```python
from build123d import *

# Parameters (mm, degrees)
ESTRUSIONE_ESTRUSIONE1_DEPTH      = 6
SCHIZZO2_R                        = 2.5
TAGLIO_ESTRUSIONE1_DEPTH          = 3
SCHIZZO3_R                        = 1.75
TAGLIO_ESTRUSIONE2_DEPTH          = 12.513144662
TAGLIO_ESTRUSIONE3_START          = -2
SCHIZZO4_R                        = 2.5
SCHIZZO4_R_2                      = 1.75
TAGLIO_ESTRUSIONE3_DEPTH          = 2
TAGLIO_ESTRUSIONE4_DEPTH          = 5
ESTRUSIONE_ESTRUSIONE2_DEPTH      = 0.2
ESTRUSIONE_ESTRUSIONE2_DEPTH_BACK = 1.2
SCHIZZO5_R                        = 2.25


with BuildPart() as part:
    # Schizzo1 → Estrusione-Estrusione1 (new body)
    with BuildSketch(Plane.XY):
        with BuildLine():
            Line((7.05, -3.5), (-7.05, -3.5))
            ThreePointArc((-7.05, -3.5), (-10.55, 0), (-7.05, 3.5))
            Line((-7.05, 3.5), (7.05, 3.5))
            ThreePointArc((7.05, 3.5), (10.55, 0), (7.05, -3.5))
        make_face()
    extrude(amount=ESTRUSIONE_ESTRUSIONE1_DEPTH)

    # Schizzo2 → Taglio-Estrusione1 (cut)
    with BuildSketch(Plane.XY.offset(6)):
        with Locations((7.05, 0)):
            Circle(SCHIZZO2_R)
    taglio_estrusione1 = extrude(amount=-TAGLIO_ESTRUSIONE1_DEPTH, mode=Mode.SUBTRACT)

    # Schizzo3 → Taglio-Estrusione2 (cut, through all)
    with BuildSketch(Plane.XY.offset(3)):
        with Locations((7.05, 0)):
            Circle(SCHIZZO3_R)
    taglio_estrusione2 = extrude(amount=-TAGLIO_ESTRUSIONE2_DEPTH, mode=Mode.SUBTRACT)

    # Schizzo4 → Taglio-Estrusione3 (cut)
    with BuildSketch(Plane(origin=(0, 0, 0), x_dir=(-1, 0, 0), z_dir=(0, 0, -1)).offset(TAGLIO_ESTRUSIONE3_START)):
        with Locations(Location((-7.05, 0, 0), (0, 0, 180))):
            Circle(SCHIZZO4_R)
        with Locations(Location((-7.05, 0, 0), (0, 0, 180))):
            Circle(SCHIZZO4_R_2, mode=Mode.SUBTRACT)
    taglio_estrusione3 = extrude(amount=TAGLIO_ESTRUSIONE3_DEPTH, mode=Mode.SUBTRACT)

    # Specchia1: Taglio-Estrusione1, Taglio-Estrusione2, Taglio-Estrusione3 across plane
    add(taglio_estrusione1.mirror(Plane(origin=(0, 0, 0), x_dir=(0, 0, 1), z_dir=(1, 0, 0))), mode=Mode.SUBTRACT)
    add(taglio_estrusione2.mirror(Plane(origin=(0, 0, 0), x_dir=(0, 0, 1), z_dir=(1, 0, 0))), mode=Mode.SUBTRACT)
    add(taglio_estrusione3.mirror(Plane(origin=(0, 0, 0), x_dir=(0, 0, 1), z_dir=(1, 0, 0))), mode=Mode.SUBTRACT)

    # Schizzo6 → Taglio-Estrusione4 (cut)
    with BuildSketch(Plane(origin=(0, 0, 0), x_dir=(-1, 0, 0), z_dir=(0, 0, -1))):
        with BuildLine():
            Line((-5.457945829, 2.75), (5.457945829, 2.75))
            ThreePointArc((5.457945829, 2.75), (3.87240083, 0), (5.457945829, -2.75))
            Line((5.457945829, -2.75), (-5.457945829, -2.75))
            ThreePointArc((-5.457945829, -2.75), (-3.87240083, 0), (-5.457945829, 2.75))
        make_face()
    extrude(amount=-TAGLIO_ESTRUSIONE4_DEPTH, mode=Mode.SUBTRACT)

    # Schizzo5 → Estrusione-Estrusione2 (add, two sides: drawn at the far end of the back side and taken through both)
    with BuildSketch(Plane.XY.offset(6).offset(-ESTRUSIONE_ESTRUSIONE2_DEPTH_BACK)):
        Circle(SCHIZZO5_R)
    extrude(amount=ESTRUSIONE_ESTRUSIONE2_DEPTH + ESTRUSIONE_ESTRUSIONE2_DEPTH_BACK)


solid = part.part
```
Check sheet for the modelled part. Datum: model origin and axes. Units: mm. A direction names the side the tool comes from. Give positions to 0.01 mm unless a question says otherwise; leave off trailing zeros. Loops run counter-clockwise (first coordinate to the right, second up) from the corner with the lowest first, then second, coordinate; pieces in that order, holes last. Notation, with made-up numbers: M -17,77.25 L 37,77.25 A23 ccw 37,96.25 Z; hole C 15,-9 d1. An arc over 180 degrees is marked long. Answer in a Markdown table with one row per item.
1) Cross-section at D-D (z = 5.5). Enter the section's corners in (x, y), plus the area to 3 significant figures.
Solutions:
| item | result |
|---|---|
| outline | M -7.05,-3.5 L 7.05,-3.5 A3.5 ccw 7.05,3.5 L -7.05,3.5 A3.5 ccw Z; hole C -7.05,0 d5; hole C 7.05,0 d5 |
| area | 97.9 mm^2 |
2) Cross-section at B-B (z = 1.75). Enter the section's corners in (x, y), plus the area to 3 significant figures.
Solutions:
| item | result |
|---|---|
| outline | M -7.05,-3.5 L 7.05,-3.5 A3.5 ccw 7.05,3.5 L -7.05,3.5 A3.5 ccw Z; hole C -7.05,0 d5; hole M -5.46,-2.75 L 5.46,-2.75 A3.18 cw 5.46,2.75 L -5.46,2.75 A3.18 cw Z; hole C 7.05,0 d5 |
| area | 50.2 mm^2 |
3) Thickness scan on line 1 (Y direction, x = 3.25, z = 3); line 2 (Y direction, x = 5, z = 2.25); line 3 (X direction, y = -0.5, z = 1). Record the ranges inside material, lowest first.
Solutions:
| item | result |
|---|---|
| line 1 | y = -3.5 to -2.75, 2.75 to 3.5 |
| line 2 | y = -3.5 to -2.75, -2.43 to 2.43, 2.75 to 3.5 |
| line 3 | x = -10.51 to -9.5, -4.6 to -3.91, 3.91 to 4.6, 9.5 to 10.51 |
4) Cross-section at A-A (x = 7.5). Enter the section's corners in (y, z).
Solutions:
| item | result |
|---|---|
| outline | M -3.47,0 L -2.46,0 L -2.46,2 L -1.69,2 L -1.69,3 L -2.46,3 L -2.46,6 L -3.47,6 Z; M 1.69,2 L 2.46,2 L 2.46,0 L 3.47,0 L 3.47,6 L 2.46,6 L 2.46,3 L 1.69,3 Z |
5) Mould release check, pull along Y, two halves, no side actions. Record for faces 4 (the face through (5, 1, 2)), 5 (the face through (10.55, 0.08, 2.96)), 6 (the face through (2.5, 0, 6)): released by +Y, released by -Y, zero draft, split by the parting line, or undercut.
Solutions:
| item | result |
|---|---|
| face 4 | undercut |
| face 5 | split by the parting line |
| face 6 | zero draft |
6) Depth check by flat-ended pin: pin 1 (1.5 mm diameter, centred on x = -6, y = 1.5, fed in from +Z); pin 2 (1.5 mm diameter, centred on x = 7.5, y = -1, fed in from -Z); pin 3 (4 mm diameter, centred on x = -7.05, y = 0, fed in from +Z); pin 4 (4 mm diameter, centred on x = -7.5, y = -1, fed in from -Z). Enter the tip coordinate at first touch or a pass-through.
Solutions:
| item | result |
|---|---|
| pin 1 | stops at z = 6 |
| pin 2 | stops at z = 2 |
| pin 3 | stops at z = 3 |
| pin 4 | stops at z = 0 |
7) Cross-section at C-C (x = 0). Enter the section's corners in (y, z).
Solutions:
| item | result |
|---|---|
| outline | M -3.5,0 L -2.75,0 L -2.75,5 L -2.25,5 L -2.25,4.8 L 2.25,4.8 L 2.25,5 L 2.75,5 L 2.75,0 L 3.5,0 L 3.5,6 L 2.25,6 L 2.25,6.2 L -2.25,6.2 L -2.25,6 L -3.5,6 Z |
8) Tool access check on faces 1 (the face through (-3, 0, 5)), 2 (the face through (9.36, -0.96, 4.52)), 3 (the face through (0, 0, 6.2)). Record the directions out of +Z, -Z, +X, -X, +Y, -Y that give a thin tool (end or side, any length) a straight path to the whole face; none if there is none.
Solutions:
| item | result |
|---|---|
| face 1 | -Z |
| face 2 | +Z |
| face 3 | +Z, +X, -X, +Y, -Y |
